Could you check a few things on this model? Use its own coordinates, in mm. Face numbers are marked on the shaded views. A direction names the side the tool comes from. Round coordinates to 2 decimals unless told otherwise and drop trailing zeros. Loops run counter-clockwise (first coordinate to the right, second up) from the corner with the lowest first, then second, coordinate; pieces in that order, holes last. Notation, with made-up numbers: (20.25, 26) -> (28.25, 26) arc R26 ccw to (28.25, 53) -> close; hole circle Ø4 at (82, 62.5). An arc over 180 degrees is marked (long way). Put each result on its own line as item: value. Start each with the question number.
1. Imagine slicing it at B-B, the plane y = 9. Please give me the cut outline in (x, z), and give its area (3 significant figures).
2. Which directions (+Z, -Z, +X, -X, +Y, -Y) give clear straight access to the entire face, cutting with the end or side of a thin tool? Please do the marked faces 4, 5, 6 and 7.
3. Imagine slicing it at C-C, the plane z = 13.25. Please give me the cut outline in (x, y) (1 decimal), and give its area (3 significant figures).
4. Imagine slicing it at A-A, the plane x = 0. Please give me the cut outline in (y, z).
5. I need wall thicknesses on line 1 (Y direction, x = 20.5, z = 13.5); line 2 (X direction, y = -0.5, z = 19.5); line 3 (X direction, y = -18, z = 15.25). Which ranges of each line are inside material? Lowest first, please. Write a range as [from, to].
6. If we mould it in two halves opening along Y, with no side actions, what happens to the marked faces 1, 2 and 3? For each: pulls with the +Y half, pulls with the -Y half, needs draft (parallel to the pull), parting line crosses it, or undercut.
7. I'm going to push flat-ended pins straight in: P1, Ø8.5, axis at x = -31, z = 16, coming from the -Y side; P2, Ø7.5, axis at x = -32.93, z = 5.93, coming from the -Y side; P3, Ø2, axis at x = -31.5, z = 6, coming from the -Y side. Where does each tip first touch, or does it pass through?
8. Imagine slicing it at D-D, the plane x = -18. Please give me the cut outline in (y, z), and give its area (3 significant figures).
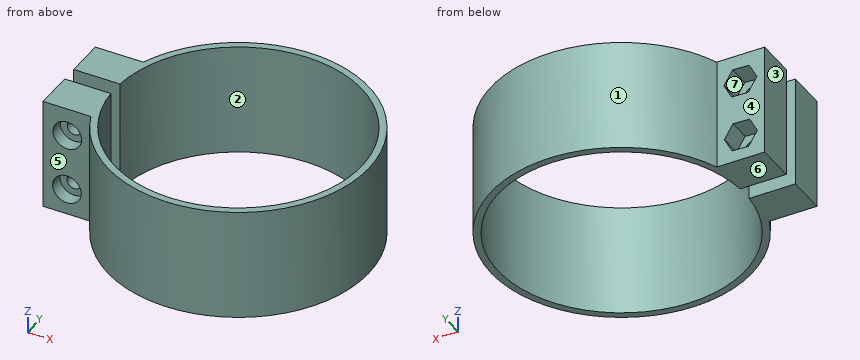
```python
from build123d import *

# Parameters (mm, degrees)
F1_DEPTH       = 25.4
F3_D           = 3.3
F3_CBORE_D     = 6.5
F3_CBORE_DEPTH = 3
F5_DEPTH       = 5


with BuildPart() as f1:
    # F0 (on Top) → F1 (new body)
    with BuildSketch(Plane.XY):
        with BuildLine():
            ThreePointArc((-27.8767053979, 1.8796), (27.94, 0), (-27.8767053979, -1.8796))
            Line((-27.8767053979, -1.8796), (-29.4676154463, -1.8796))
            Line((-29.4676154463, -1.8796), (-38.3576154463, -1.8796))
            Line((-38.3576154463, -1.8796), (-38.3576154463, -10.7696))
            Line((-38.3576154463, -10.7696), (-29.4676154463, -10.7696))
            Line((-29.4676154463, -10.7696), (-27.4934350726, -10.7696))
            ThreePointArc((-27.4934350726, -10.7696), (29.5275, 0), (-27.4934350726, 10.7696))
            Line((-27.4934350726, 10.7696), (-29.4676154463, 10.7696))
            Line((-29.4676154463, 10.7696), (-38.3576154463, 10.7696))
            Line((-38.3576154463, 10.7696), (-38.3576154463, 1.8796))
            Line((-38.3576154463, 1.8796), (-29.4676154463, 1.8796))
            Line((-29.4676154463, 1.8796), (-27.8767053979, 1.8796))
        make_face()
    extrude(amount=F1_DEPTH)

    # F3 (through all)
    with Locations(Plane.XZ.offset(10.7696)):
        with Locations((-32.8522585332, 18.9988464117), (-32.9255252594, 5.9281084687)):
            CounterBoreHole(F3_D / 2, F3_CBORE_D / 2, F3_CBORE_DEPTH)

    # F4 (on face) → F5 (cut)
    with BuildSketch(Plane(origin=(0, 10.7696, 0), x_dir=(-1, 0, 0), z_dir=(0, 1, 0))):
        Polygon((34.6081861546, 15.6860156038), (36.599217982, 18.8631089351), (34.8432903606, 22.175939743), (31.0963309118, 22.3116772196), (29.1052990845, 19.1345838883), (30.8612267059, 15.8217530804), align=None)
        Polygon((36.7005912762, 5.7845558547), (34.9446636548, 9.0973866626), (31.197704206, 9.2331241392), (29.2066723786, 6.0560308079), (30.9626, 2.7432), (34.7095594488, 2.6074625234), align=None)
    extrude(amount=-F5_DEPTH, mode=Mode.SUBTRACT)


solid = f1.part
```
Entries:
1. outline: (-38.36, 0) -> (-26.45, 0) -> (-26.45, 25.4) -> (-38.36, 25.4) -> close; (26.45, 0) -> (28.12, 0) -> (28.12, 25.4) -> (26.45, 25.4) -> close; hole (-36.7, 5.78) -> (-34.71, 2.61) -> (-30.96, 2.74) -> (-29.21, 6.06) -> (-31.2, 9.23) -> (-34.94, 9.1) -> close; hole (-36.6, 18.86) -> (-34.61, 15.69) -> (-30.86, 15.82) -> (-29.11, 19.13) -> (-31.1, 22.31) -> (-34.84, 22.18) -> close
1. area: 272 mm^2
2. face 4: +Z, -Z, -X, +Y
2. face 5: +Z, -Z, -X, -Y
2. face 6: -Z, +X, -X, +Y, -Y
2. face 7: +Y
3. outline: (-38.4, -10.8) -> (-27.5, -10.8) arc R29.5 ccw (long way) to (-27.5, 10.8) -> (-38.4, 10.8) -> (-38.4, 1.9) -> (-27.9, 1.9) arc R27.9 cw (long way) to (-27.9, -1.9) -> (-38.4, -1.9) -> close
3. area: 452 mm^2
4. outline: (-29.53, 0) -> (-27.94, 0) -> (-27.94, 25.4) -> (-29.53, 25.4) -> close; (27.94, 0) -> (29.53, 0) -> (29.53, 25.4) -> (27.94, 25.4) -> close
5. line 1: [-21.25, -18.98], [18.98, 21.25]
5. line 2: [27.94, 29.52]
5. line 3: [-23.41, -21.37], [21.37, 23.41]
6. face 1: parting line crosses it
6. face 2: undercut
6. face 3: needs draft
7. P1: y = -12.5
7. P2: y = -10.77
7. P3: y = -7.77
8. outline: (-23.41, 0) -> (-21.37, 0) -> (-21.37, 25.4) -> (-23.41, 25.4) -> close; (21.37, 0) -> (23.41, 0) -> (23.41, 25.4) -> (21.37, 25.4) -> close
8. area: 104 mm^2
